Geometry: final body of the model. Coordinates: model frame, mm. Give positions to 0.01 mm unless a question says otherwise; leave off trailing zeros. Order: outer loops, then holes, each group sorted by start corner. A loop starts at its lowest first (then second) coordinate and runs counter-clockwise, first axis right, second up. Notation, with made-up numbers: (82.25, 25.5) - (127.25, 25.5) arc R18 ccw to (127.25, 34.5) - close; hole circle Ø1 at (-32, -16). An arc over 180 degrees is marked (long way). Put each result on its own line as item: value. Start each with the question number.
1. Mould query, pull axis Y, two halves, no side actions, for faces 1 (the cylindrical face through (590.9, 701.27, 779.67)), 2 (the flat face through (573, 587, 1250.979)), 3 (the flat face through (573, -76.2, 625)). Classes: pulls with the +Y half, pulls with the -Y half, needs draft (parallel to the pull), parting line crosses it, or undercut.
2. Section C-C on x = 481. Return the cut outline in (y, z).
3. Ray query, line 1 along Z through (x, y) = (378, 596); line 2 along Y through (x, z) = (178.5, 682.5); line 3 along Y through (x, z) = (968.5, 442). Return the intervals inside material, ascending. Write a range as from..to.
4. Section B-B on z = 557. Return the cut outline in (x, y), plus the area to 3 significant figures.
5. Section A-A on y = 596.9. Return the cut outline in (x, z), plus the area to 3 significant figures.
from build123d import *

# Parameters (mm, degrees)
F0_W      = 1270
F0_H      = 1270
F1_DEPTH  = 76.2
F1_FACE_W = 1270
F1_FACE_H = 1270
F2_DEPTH  = 1270
F3_R      = 194.135033
F4_DEPTH  = 40.64
F4_FACE_R = 194.135033
F5_DEPTH  = 1397


with BuildPart() as f1:
    # F0 (on Front) → F1 (new body)
    with BuildSketch(Plane.XZ):
        with Locations((582.012902, 615.979133)):
            Rectangle(F0_W, F0_H)
    extrude(amount=F1_DEPTH)

    # F1_face (on face) → F2 (join)
    with BuildSketch(Plane(origin=(582.012902, 0, 615.979133), x_dir=(1, 0, 0), z_dir=(0, 1, 0))):
        Rectangle(F1_FACE_W, F1_FACE_H)
    extrude(amount=F2_DEPTH)

    # F3 (on face) → F4 (join)
    with BuildSketch(Plane.YZ.offset(1217.012902)):
        with Locations((596.9, 615.979133)):
            Circle(F3_R)
    extrude(amount=F4_DEPTH)

    # F4_face (on face) → F5 (cut)
    with BuildSketch(Plane(origin=(1257.652902, 596.9, 615.979133), x_dir=(0, 1, 0), z_dir=(1, 0, 0))):
        Circle(F4_FACE_R)
    extrude(amount=-F5_DEPTH, mode=Mode.SUBTRACT)


solid = f1.part
Resolved:
1. face 1: undercut
1. face 2: needs draft
1. face 3: pulls with the -Y half
2. outline: (-76.2, -19.02) - (1270, -19.02) - (1270, 1250.98) - (-76.2, 1250.98) - close; hole circle Ø388.27 at (596.9, 615.98)
3. line 1: -19.02..421.85, 810.11..1250.98
3. line 2: -76.2..414.52, 779.28..1270
3. line 3: -76.2..510.76, 683.04..1270
4. outline: (-52.99, -76.2) - (1217.01, -76.2) - (1217.01, 411.94) - (-52.99, 411.94) - close; (-52.99, 781.86) - (1217.01, 781.86) - (1217.01, 1270) - (-52.99, 1270) - close
4. area: 1,240,000 mm^2
5. outline: (-52.99, -19.02) - (1217.01, -19.02) - (1217.01, 421.84) - (-52.99, 421.84) - close; (-52.99, 810.11) - (1217.01, 810.11) - (1217.01, 1250.98) - (-52.99, 1250.98) - close
5. area: 1,120,000 mm^2
